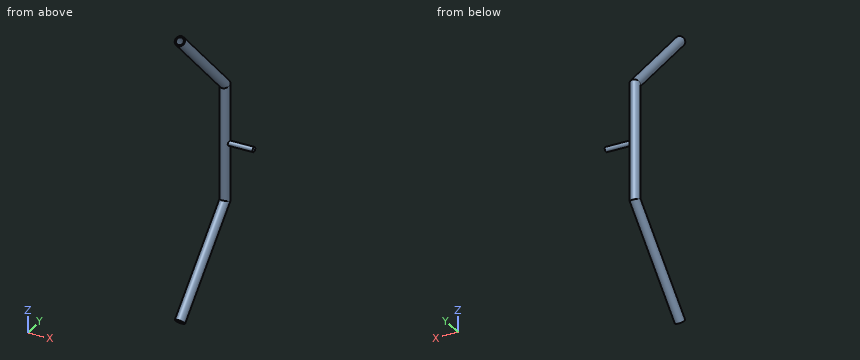
```python
from build123d import *

# Parameters (mm, degrees)
SWEEP1_PROFILE_R     = 12.7
CUT_SWEEP1_PROFILE_R = 9.525
SKETCH19_R           = 6.35
BOSS_EXTRUDE1_DEPTH  = 76.2


with BuildPart() as part:
    # Sweep1: sweep along a path in Sketch2
    with BuildLine(Plane(origin=(0, 0, 0), x_dir=(0, 0, -1), z_dir=(1, 0, 0))) as sweep1_path:
        Line((-248.182278836, -217.015933946), (-32.65613193, -1.489787041))
        Line((-32.65613193, -1.489787041), (272.14386807, -1.489787041))
        Line((272.14386807, -1.489787041), (487.670014975, -217.015933946))
    # Sweep1 profile (on start of the path) → Sweep1 (sweep)
    with BuildSketch(Plane(origin=(0, -217.015933946, 248.182278836), x_dir=(0, 0.707106781, 0.707106781), z_dir=(0, 0.707106781, -0.707106781))):
        Circle(SWEEP1_PROFILE_R)
    sweep(path=sweep1_path.line, transition=Transition.RIGHT)

    # Cut-Sweep1: sweep along a path in Sketch2_2
    with BuildLine(Plane(origin=(0, 0, 0), x_dir=(0, 0, -1), z_dir=(1, 0, 0))) as cut_sweep1_path:
        Line((-248.182278836, -217.015933946), (-32.65613193, -1.489787041))
        Line((-32.65613193, -1.489787041), (272.14386807, -1.489787041))
        Line((272.14386807, -1.489787041), (487.670014975, -217.015933946))
    # Cut-Sweep1 profile (on start of the path) → Cut-Sweep1 (sweep, cut)
    with BuildSketch(Plane(origin=(0, -217.015933946, 248.182278836), x_dir=(0, 0.707106781, 0.707106781), z_dir=(0, 0.707106781, -0.707106781))):
        Circle(CUT_SWEEP1_PROFILE_R)
    sweep(path=cut_sweep1_path.line, transition=Transition.RIGHT, mode=Mode.SUBTRACT)

    # Sketch19 → Boss-Extrude1 (add)
    with BuildSketch(Plane(origin=(0, 0, 0), x_dir=(0, 0, -1), z_dir=(1, 0, 0))):
        with Locations((119.74386807, -1.489787041)):
            Circle(SKETCH19_R)
    extrude(amount=BOSS_EXTRUDE1_DEPTH)


solid = part.part
```
Verification items for the finished model (mm, model axes). Round coordinates to 2 decimals unless told otherwise and drop trailing zeros. Write each loop counter-clockwise with the first axis right and the second up, starting at its lowest first coordinate (ties: lowest second). Pieces come first, ordered by that corner, then holes.
1. Scan lines: L1, parallel to Z at x = 0.5, y = -108.5; L2, parallel to Z at x = -8, y = -65; L3, parallel to X at y = -108.5, z = 147. Record each from-to range of solid material in increasing order.
2. Gauge pin test, flat ends, axial feed: P1, Ø6, axis at y = -88, z = -378.5, coming from the -X side; P2, Ø15, axis at x = 0, y = -1.49, coming from the -Z side; P3, Ø10, axis at x = 12, z = -108, coming from the -Y side. Record the tip position at first contact, or that the pin passes through.
3. Section check A-A on z = -73. Enter the section's corners in (x, y) (3 decimals), plus the area to 3 significant figures.
4. Section check B-B on y = -128. State how many separate pieces and enclosed holes the cut face has, plus the area to 3 significant figures.
5. Section check C-C on x = 30. Enter the section's corners in (y, z).
Answer:
1. L1: z = -397.1 to -392.61, -365.7 to -361.21, 121.72 to 126.21, 153.12 to 157.61
1. L2: z = -349.6 to -342.97, -328.34 to -321.7, 82.22 to 88.86, 103.48 to 110.12
1. L3: x = -11.59 to -7.99, 7.99 to 11.59
2. P1: stops at x = -6.29
2. P2: stops at z = -297.6
2. P3: stops at y = -12.09
3. outline: circle Ø25.4 at (0, -1.49); hole circle Ø19.05 at (0, -1.49)
3. area: 222 mm2
4. separate pieces: 2
4. enclosed holes: 2
4. area: 627 mm2
5. outline: circle Ø12.7 at (-1.49, -119.74)
